from build123d import *

# Parameters (mm, degrees)
PAD002_DEPTH    = 3
POCKET001_DEPTH = 5
PAD003_DEPTH    = 10
FILLET_R        = 8
FILLET001_R     = 8
FILLET002_R     = 8
PAD004_DEPTH    = 3
SKETCH007_W     = 2
SKETCH007_H     = 4
SKETCH007_W_2   = 4
SKETCH007_H_2   = 2
PAD005_DEPTH    = 6
SKETCH008_R     = 5.3
POCKET002_DEPTH = 5


with BuildPart() as part:
    # Sketch003 → Pad002 (new body)
    with BuildSketch(Plane.XY.offset(3.2)):
        Polygon((-63.6396103068, 90.5096679919), (-12.4299423149, 39.3), (-0.7, 39.3), (-0.7, 0.7), (-39.3, 0.7), (-39.3, 12.4299423149), (-90.5096679919, 63.6396103068), (-103.6396103068, 63.6396103068), (-103.6396103068, 103.6396103068), (-63.6396103068, 103.6396103068), align=None)
    extrude(amount=PAD002_DEPTH)

    # Sketch004 (on Face12 of Pad002) → Pocket001 (cut)
    with BuildSketch(Plane.XY.offset(6.2)):
        Polygon((-95.660425587, 75.8614357137), (-91.4177848998, 80.1040764009), (-87.1751442127, 75.8614357137), (-91.4177848998, 71.6187950266), align=None)
        Polygon((-75.8614357137, 87.1751442127), (-80.1040764009, 91.4177848998), (-75.8614357137, 95.660425587), (-71.6187950266, 91.4177848998), align=None)
        Polygon((-87.1751442127, 91.4177848998), (-91.4177848998, 87.1751442127), (-95.660425587, 91.4177848998), (-91.4177848998, 95.660425587), align=None)
        Polygon((-75.8614357137, 80.1040764009), (-80.1040764009, 75.8614357137), (-75.8614357137, 71.6187950266), (-71.6187950266, 75.8614357137), align=None)
    extrude(amount=-POCKET001_DEPTH, mode=Mode.SUBTRACT)

    # Sketch005 (on Face5 of Pocket001) → Pad003 (join)
    with BuildSketch(Plane.XY.offset(6.2)):
        with BuildLine():
            ThreePointArc((-67.3761543395, 78.6898628385), (-95.660425587, 95.660425587), (-78.6898628385, 67.3761543395))
            Line((-78.6898628385, 67.3761543395), (-78.1075396069, 65.4628065786))
            ThreePointArc((-65.4628065786, 78.1075396069), (-97.0746391493, 97.0746391493), (-78.1075396069, 65.4628065786))
            Line((-67.3761543395, 78.6898628385), (-65.4628065786, 78.1075396069))
        make_face()
    extrude(amount=PAD003_DEPTH)

    # Fillet
    fillet_edges = [part.edges().sort_by_distance(p)[0] for p in [
        (-103.63961, 63.63961, 4.7),
    ]]
    fillet(fillet_edges, radius=FILLET_R)

    # Fillet001
    fillet001_edges = [part.edges().sort_by_distance(p)[0] for p in [
        (-103.63961, 103.63961, 4.7),
    ]]
    fillet(fillet001_edges, radius=FILLET001_R)

    # Fillet002
    fillet002_edges = [part.edges().sort_by_distance(p)[0] for p in [
        (-63.63961, 103.63961, 4.7),
    ]]
    fillet(fillet002_edges, radius=FILLET002_R)

    # Sketch006 (on Face31 of Fillet002) → Pad004 (join)
    with BuildSketch(Plane.XY.offset(6.2)):
        Polygon((-80.6101730553, 65.0538238692), (-78.4888527117, 67.1751442127), (-42.4264068712, 31.1126983722), (-44.5477272148, 28.9913780286), align=None)
        Polygon((-67.1751442128, 78.4888527117), (-65.0538238692, 80.6101730553), (-28.9913780286, 44.5477272148), (-31.1126983722, 42.4264068711), align=None)
    extrude(amount=PAD004_DEPTH)

    # Sketch007 (on Face31 of Pad004) → Pad005 (join)
    with BuildSketch(Plane.XY.offset(6.2)):
        with Locations((-83.6396103068, 98.6396103068)):
            Rectangle(SKETCH007_W, SKETCH007_H)
        with Locations((-98.6396103068, 83.6396103068)):
            Rectangle(SKETCH007_W_2, SKETCH007_H_2)
        with Locations((-68.6414357137, 83.6396103068)):
            Rectangle(SKETCH007_W_2, SKETCH007_H_2)
        with Locations((-83.6396103068, 68.6414357137)):
            Rectangle(SKETCH007_W, SKETCH007_H)
    extrude(amount=PAD005_DEPTH)

    # Sketch008 (on Face31 of Pad005) → Pocket002 (cut)
    with BuildSketch(Plane.XY.offset(6.2)):
        with Locations((-30, 30)):
            Circle(SKETCH008_R)
        with Locations((-10, 30)):
            Circle(SKETCH008_R)
        with Locations((-30, 10)):
            Circle(SKETCH008_R)
        with Locations((-10, 10)):
            Circle(SKETCH008_R)
    extrude(amount=-POCKET002_DEPTH, mode=Mode.SUBTRACT)


solid = part.part
Work out the finished part from the listing and answer in its coordinate system (mm). A direction names the side the tool comes from. Give positions to 0.01 mm unless a question says otherwise; leave off trailing zeros. Loops run counter-clockwise (first coordinate to the right, second up) from the corner with the lowest first, then second, coordinate; pieces in that order, holes last. Notation, with made-up numbers: (9.5, 39.25) -> (58.5, 39.25) arc R21 ccw to (58.5, 56.25) -> close; hole circle Ø11 at (-6, -37.75). An arc over 180 degrees is marked (long way). Use a Markdown table: item, result. Add a question column.
1) Which of the six approach directions +Z, -Z, +X, -X, +Y, -Y give full straight-line access (tool end or side, diameter ignored) to faces 1 (the flat face through (-82.64, 69, 9)), 2 (the flat face through (-39.3, 6, 5)), 3 (the flat face through (-73.71, 77.95, 4.72))?
2) The part is cut by section A-A, the plane x = -10. Determine the outline of the cut face in (y, z), plus the area to 3 significant figures.
3) Consider line 1 along Y through (x, z) = (-10, 4.65); line 2 along Y through (x, z) = (-9, 4); line 3 along Z through (x, y) = (-84.5, 82). Determine where each line is inside the solid, lowest interval first.
4) The part is cut by section C-C, the plane x = -58.5. Determine the outline of the cut face in (y, z), plus the area to 3 significant figures.
5) Each of these flat-tipped pins is pushed along its axis until it touches: P1, Ø3, axis at x = -68.5, z = 10, coming from the +Y side; P2, Ø1.5, axis at y = 93.5, z = 5, coming from the +X side; P3, Ø1.2, axis at x = -69, z = 9.5, coming from the -Y side; P4, Ø9.5, axis at x = -30, y = 30, coming from the +Z side. Where does it stop, or does it pass through?
6) For a pull along Y with two mould halves and no side action, classify faces 4 (the flat face through (-99, 84.64, 9)), 5 (the flat face through (-38.39, 65.26, 4.68)), 6 (the flat face through (-64.55, 37.68, 4.68)) as +Y half, -Y half, draft (parallel to the pull), parting line (faces both ways), or undercut.
7) The part is cut by section B-B, the plane y = 10. Determine the outline of the cut face in (x, z), plus the area to 3 significant figures.
8) The part is cut by section D-D, the plane y = 58. Determine the outline of the cut face in (x, z).
Reported:
| question | item | result |
|---|---|---|
| 1 | face 1 | +Z |
| 1 | face 2 | +Z, -Z, -X, -Y |
| 1 | face 3 | +Z, -Z |
| 2 | outline | (0.7, 3.2) -> (4.7, 3.2) -> (4.7, 6.2) -> (0.7, 6.2) -> close; (15.3, 3.2) -> (24.7, 3.2) -> (24.7, 6.2) -> (15.3, 6.2) -> close; (35.3, 3.2) -> (39.3, 3.2) -> (39.3, 6.2) -> (35.3, 6.2) -> close |
| 2 | area | 52.2 mm^2 |
| 3 | line 1 | y = 0.7 to 4.7, 15.3 to 24.7, 35.3 to 39.3 |
| 3 | line 2 | y = 0.7 to 4.8, 15.2 to 24.8, 35.2 to 39.3 |
| 3 | line 3 | z = 3.2 to 6.2 |
| 4 | outline | (31.63, 3.2) -> (85.37, 3.2) -> (85.37, 6.2) -> (74.06, 6.2) -> (74.06, 9.2) -> (69.81, 9.2) -> (69.81, 6.2) -> (47.19, 6.2) -> (47.19, 9.2) -> (42.94, 9.2) -> (42.94, 6.2) -> (31.63, 6.2) -> close |
| 4 | area | 187 mm^2 |
| 5 | P1 | stops at y = 96.87 |
| 5 | P2 | stops at x = -63.64 |
| 5 | P3 | stops at y = 52.92 |
| 5 | P4 | passes through |
| 6 | face 4 | undercut |
| 6 | face 5 | +Y half |
| 6 | face 6 | -Y half |
| 7 | outline | (-39.3, 3.2) -> (-35.3, 3.2) -> (-35.3, 6.2) -> (-39.3, 6.2) -> close; (-24.7, 3.2) -> (-15.3, 3.2) -> (-15.3, 6.2) -> (-24.7, 6.2) -> close; (-4.7, 3.2) -> (-0.7, 3.2) -> (-0.7, 6.2) -> (-4.7, 6.2) -> close |
| 7 | area | 52.2 mm^2 |
| 8 | outline | (-84.87, 3.2) -> (-31.13, 3.2) -> (-31.13, 6.2) -> (-42.44, 6.2) -> (-42.44, 9.2) -> (-46.69, 9.2) -> (-46.69, 6.2) -> (-69.31, 6.2) -> (-69.31, 9.2) -> (-73.56, 9.2) -> (-73.56, 6.2) -> (-84.87, 6.2) -> close |
